Geometry: final body of the model. Coordinates: model frame, mm. Face numbers are marked on the shaded views. A direction names the side the tool comes from. Coordinates: 2 decimals unless noted, no trailing zeros. Write each loop counter-clockwise with the first axis right and the second up, starting at its lowest first coordinate (ties: lowest second). Pieces come first, ordered by that corner, then holes.
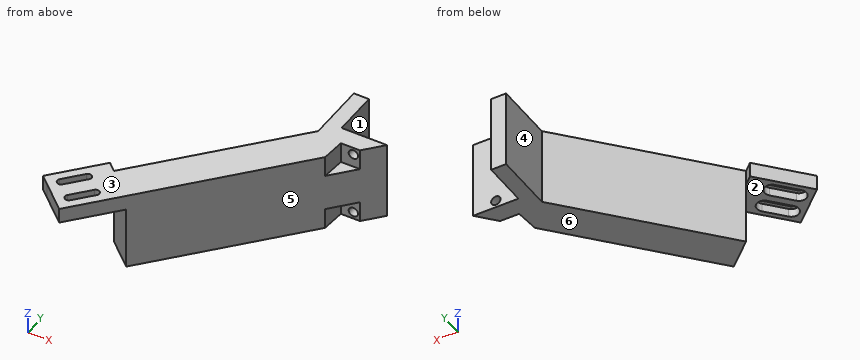
Autodesk Inventor part; units mm, degrees
ref_plane "Work Plane2" through (-4.445, -9.144, -33.02) normal (0, 0, -1) x (0, 1, 0)
ref_plane "YZ Plane" through (0, 0, 0) normal (1, 0, 0) x (0, 1, 0)
ref_plane "XZ Plane" through (0, 0, 0) normal (0, 1, 0) x (-1, 0, 0)
ref_plane "Work Plane1" through (0, 0, 0) normal (0, 0, 1) x (1, 0, 0)
sketch "Sketch1" plane through (0, 0, 0) normal (0, 0, 1) x (1, 0, 0)
  line L0 (4.129202, -9.5377) -> (6.406797, -9.5377) construction
  line L1 (9.525, -8.41296) -> (9.525, -7.435497) construction
  line L2 (-6.406797, 9.5123) -> (-4.129202, 9.5123) construction
  line L3 (-9.525, 4.116502) -> (-9.525, 6.394097) construction
  line L4 (9.314549, -9.373063) -> (-73.965447, -101.864868) construction
  line L5 (9.166309, -9.5377) -> (-73.965447, -101.864868)
  line L6 (-73.965447, -101.864868) -> (-85.121243, -91.820144)
  line L7 (6.33881, 9.756536) -> (-85.121243, -91.820144) construction
  line L8 (9.166309, -9.5377) -> (-9.997679, -9.5377)
  line L9 (-9.997679, -9.5377) -> (-9.997679, 9.756536)
  line L10 (-9.997679, 9.756536) -> (-16.347679, 9.756536)
  line L11 (-16.347679, 9.756536) -> (-16.347679, -15.439362)
  line L12 (-16.347679, -15.439362) -> (-85.121243, -91.820144)
  point P0 (0, 0)
  dimension "d0" = 124.46
  dimension "d1" = 48
  dimension "d5" = 6.35
ref_plane "Work Plane2" through (-4.445, -9.144, -33.02) normal (0, 0, -1) x (0, 1, 0)
extrude "Extrusion1" add sketch "Sketch1" against normal up to surface (33.02 mm away)
sketch "Sketch2" plane through (-73.965447, -101.864868, -33.02) normal (-0.6691306, -0.7431448, 0) x (0.7431448, -0.6691306, 0)
  line L0 (0, 33.02) -> (0, 0)
  line L1 (-15.011605, 33.02) -> (-15.011605, 0)
  line L2 (0, 0) -> (-15.011605, 0)
  line L3 (-15.011605, 0) -> (-15.011605, 26.67)
  line L4 (-15.011605, 26.67) -> (0, 26.67)
  line L5 (0, 26.67) -> (0, 0)
  line L6 (-15.011605, 33.02) -> (0, 33.02)
  point P0 (-13.193862, 33.02)
  dimension "d19" = 6.35
extrude "Extrusion2" cut sketch "Sketch2" against normal blind 25.4 contours L0 L2 L1 L4
sketch "Sketch3" plane through (-73.965447, -101.864868, -6.35) normal (0, 0, -1) x (-0.7431448, 0.6691306, 0)
  line L0 (19.8882, 12.0904) -> (19.8882, 3.175) construction
  line L1 (0, 25.4) -> (15.011605, 25.4) construction
  line L2 (15.011605, 0) -> (0, 0) construction
  line L3 (0, 0) -> (19.8882, 0) construction
  line L4 (19.8882, 0) -> (19.8882, 25.4) construction
  line L5 (19.8882, 25.4) -> (0, 25.4) construction
  line L6 (0, 25.4) -> (0, 0) construction
  line L7 (15.011605, 0) -> (19.8882, 0)
  line L8 (19.8882, 0) -> (19.8882, 25.4)
  line L9 (19.8882, 25.4) -> (15.011605, 25.4)
  line L10 (15.011605, 25.4) -> (15.011605, 0)
  point P0 (13.193862, 125.192894)
extrude "Extrusion3" add sketch "Sketch3" against normal up to surface (6.35 mm away)
sketch "Sketch4" plane through (0, 0, 0) normal (0, 0, 1) x (1, 0, 0)
  line L0 (-88.74526, -88.557064) -> (-71.749342, -69.681186) construction
  line L1 (-73.965447, -101.864868) -> (9.166309, -9.5377) construction
  line L2 (-74.314967, -94.50927) -> (-67.5166, -86.958918) construction
  line L3 (-73.965447, -101.864868) -> (-56.969529, -82.988989) construction
  line L4 (-73.965447, -101.864868) -> (-88.74526, -88.557064) construction
  line L5 (-81.390199, -88.138702) -> (-74.591832, -80.588351) construction
  line L6 (-74.314967, -94.50927) -> (-67.5166, -86.958918) construction
  line L7 (-73.144662, -95.563017) -> (-66.346296, -88.012665)
  line L8 (-68.686904, -85.905171) -> (-75.485271, -93.455523)
  arc A0 (-75.485271, -93.455523) -> (-73.144662, -95.563017) centre (-74.314967, -94.50927) ccw
  arc A1 (-66.346296, -88.012665) -> (-68.686904, -85.905171) centre (-67.5166, -86.958918) ccw
  line L9 (-81.390199, -88.138702) -> (-74.591832, -80.588351) construction
  line L10 (-80.219894, -89.192449) -> (-73.421527, -81.642098)
  line L11 (-75.762136, -79.534604) -> (-82.560503, -87.084955)
  arc A2 (-82.560503, -87.084955) -> (-80.219894, -89.192449) centre (-81.390199, -88.138702) ccw
  arc A3 (-73.421527, -81.642098) -> (-75.762136, -79.534604) centre (-74.591832, -80.588351) ccw
  point P0 (0, 0)
  point P1 (-70.915783, -90.734094)
  point P2 (-77.991015, -84.363527)
  dimension "d37" = 10.16
  dimension "d38" = 5.1816
  dimension "d39" = 5.2324
  dimension "d40" = 9.52066
  dimension "d41" = 3.1496
  dimension "d42" = 3.1496
extrude "Extrusion4" cut sketch "Sketch4" against normal through all
sketch "Sketch6" plane through (-9.997679, -9.5377, 0) normal (0, 1, 0) x (1, 0, 0)
  arc A0 (9.506526, 4.79213) -> (10.740649, 4.300966) centre (9.523849, 3.039616) ccw construction
  arc A1 (9.506526, 31.732899) -> (10.740649, 31.241734) centre (9.523849, 29.980384) ccw construction
  circle A2 centre (9.523849, 29.980384) radius 1.9685
  circle A3 centre (9.523849, 3.039616) radius 1.9685
  point P0 (9.997679, 0)
  dimension "d24" = 3.937
  dimension "d25" = 3.937
extrude "Extrusion6" cut sketch "Sketch6" against normal through all
sketch "Sketch7" plane through (9.166309, -9.5377, 0) normal (0.7431448, -0.6691306, 0) x (0, 0, -1)
  line L0 (33.02, -98.838459) -> (33.02, 0) construction
  line L1 (33.02, -9.525) -> (0, -9.525) construction
  point P0 (0, 0.954435)
sketch "Sketch8" plane through (9.166309, -9.5377, -33.02) normal (0, 0, -1) x (-1, 0, 0)
  line L0 (11.608639, 0) -> (11.608639, -12.892699) construction
  line L1 (66.135838, -73.451289) -> (0, 0) construction
  line L2 (11.608639, -7.62) -> (6.861079, -7.62) construction
  line L3 (0, 0) -> (19.163987, 0) construction
  line L4 (7.671639, 0) -> (7.671639, -8.520218) construction
  line L5 (14.910639, 0) -> (14.910639, -14.251905) construction
  line L6 (6.861079, -7.62) -> (14.910639, -7.62)
  line L7 (83.131755, -92.327168) -> (0, 0)
  line L8 (15.69062, -17.426199) -> (6.861079, -7.62)
  line L9 (15.69062, -17.426199) -> (14.910639, -7.62)
  point P0 (9.166309, 9.5377)
  dimension "d28" = 7.62
  dimension "d29" = 3.302
extrude "Extrusion7" cut sketch "Sketch8" against normal blind 8.763
sketch "Sketch9" plane through (0, 0, 0) normal (0, 0, 1) x (1, 0, 0)
  line L0 (2.30523, -17.1577) -> (-5.74433, -17.1577) construction
  line L1 (-5.74433, -17.1577) -> (-6.524312, -26.963899) construction
  line L2 (2.30523, -17.1577) -> (-6.524312, -26.963899)
  line L3 (-73.965447, -101.864868) -> (9.166309, -9.5377)
  line L4 (2.30523, -17.1577) -> (-5.74433, -17.1577)
  line L5 (-5.2705, -26.963899) -> (-5.2705, -17.1577)
  point P0 (0, 0)
sketch "Sketch9 outline for Extrusion8" plane through (0, 0, 0) normal (0, 0, 1) x (1, 0, 0)
  line L0 (-6.524312, -26.963899) -> (2.30523, -17.1577)
  line L1 (-5.74433, -17.1577) -> (-6.524312, -26.963899)
  line L2 (2.30523, -17.1577) -> (-5.74433, -17.1577)
extrude "Extrusion8" cut sketch "Sketch9 outline for Extrusion8" against normal blind 8.763
sketch "Sketch10" plane through (9.166309, -9.5377, -33.02) normal (0, 0, -1) x (-1, 0, 0)
  line L0 (25.513987, -5.901662) -> (77.291634, -63.406565)
  line L1 (51.797758, -35.092747) -> (40.641962, -45.137471)
  line L2 (66.135838, -73.451289) -> (15.69062, -17.426199) construction
  line L3 (40.913229, -45.438744) -> (36.5125, -40.551239) construction
  line L4 (66.135838, -73.451289) -> (77.291634, -63.406565) construction
  point P0 (9.166309, 9.5377)
  dimension "d34" = 38.1
sketch "Sketch11" plane through (-73.965447, -101.864868, -6.35) normal (0, 0, -1) x (-0.7431448, 0.6691306, 0)
  arc A0 (3.6068, 5.2324) -> (6.7564, 5.2324) centre (5.1816, 5.2324) ccw construction
  arc A1 (6.7564, 15.3924) -> (3.6068, 15.3924) centre (5.1816, 15.3924) ccw construction
  line L0 (5.1816, 5.2324) -> (5.1816, 15.3924) construction
  arc A2 (13.127463, 5.2324) -> (16.277063, 5.2324) centre (14.702263, 5.2324) ccw construction
  arc A3 (16.277063, 15.3924) -> (13.127463, 15.3924) centre (14.702263, 15.3924) ccw construction
  line L1 (14.702263, 5.2324) -> (14.702263, 15.3924) construction
  line L2 (14.702263, 5.2324) -> (14.702263, 15.3924) construction
  line L3 (17.877263, 5.2324) -> (17.877263, 15.3924)
  line L4 (11.527263, 15.3924) -> (11.527263, 5.2324)
  arc A4 (11.527263, 5.2324) -> (17.877263, 5.2324) centre (14.702263, 5.2324) ccw
  arc A5 (17.877263, 15.3924) -> (11.527263, 15.3924) centre (14.702263, 15.3924) ccw
  line L5 (5.1816, 5.2324) -> (5.1816, 15.3924) construction
  line L6 (8.3566, 5.2324) -> (8.3566, 15.3924)
  line L7 (2.0066, 15.3924) -> (2.0066, 5.2324)
  arc A6 (2.0066, 5.2324) -> (8.3566, 5.2324) centre (5.1816, 5.2324) ccw
  arc A7 (8.3566, 15.3924) -> (2.0066, 15.3924) centre (5.1816, 15.3924) ccw
  point P0 (13.193862, 125.192894)
  point P1 (14.702263, 10.3124)
  point P2 (5.1816, 10.3124)
  dimension "d43" = 6.35
  dimension "d44" = 6.35
extrude "Extrusion9" cut sketch "Sketch11" against normal blind 3.556
properties part number "arm stop 48 degree whole"
Item 1: Set-up query: the marked faces 1, 2 and 3. Return all of +Z, -Z, +X, -X, +Y, -Y with unobstructed straight access to the full face (end or side cutting, diameter ignored); none if empty.
Derived:
face 1: +Z, -Z, +X, +Y
face 2: -Z, -X, -Y
face 3: +Z, +X, -X, +Y, -Y
Item 2: Section A-A, the plane z = -13.5. Output: boundary loops of the cut face in (x, y), plus the area to 3 significant figures.
Derived:
outline: (-68.12, -72.94) - (-56.97, -82.99) - (9.17, -9.54) - (-10, -9.54) - (-10, 9.76) - (-16.35, 9.76) - (-16.35, -15.44) - close
area: 1,520 mm2
Item 3: Section D-D, the plane y = -38. Output: boundary loops of the cut face in (x, z), plus the area to 3 significant figures.
Derived:
outline: (-36.66, -33.02) - (-16.46, -33.02) - (-16.46, 0) - (-36.66, 0) - close
area: 667 mm2
Item 4: Pin query (flat end, axial travel): pin 1 (12 mm diameter, centred on y = -2.5, z = -22.5, fed in from -X); pin 2 (4 mm diameter, centred on x = -1.5, z = -4.5, fed in from -Y); pin 3 (1 mm diameter, centred on y = -25.5, z = -27.5, fed in from -X). Return the tip coordinate at first contact, or that it passes through.
Derived:
pin 1: stops at x = -16.35
pin 2: stops at y = -17.16
pin 3: stops at x = -25.86
Item 5: Section C-C, the plane y = -25.5. Output: boundary loops of the cut face in (x, z), plus the area to 3 significant figures.
Derived:
outline: (-25.41, -33.02) - (-6.41, -33.02) - (-6.41, -24.26) - (-5.21, -24.26) - (-5.21, -8.76) - (-6.41, -8.76) - (-6.41, 0) - (-25.41, 0) - close
area: 646 mm2
Item 6: Material intervals for probe 1 along X at (y, z) = (3.5, -5); probe 2 along Z at (x, y) = (-70.5, -95.5); probe 3 along Y at (x, z) = (2, -1.5), sorted ascending.
Derived:
probe 1: x = -16.35 to -10
probe 2: z = -6.35 to 0
probe 3: y = -17.16 to -9.54
Item 7: Section B-B, the plane x = -4. Output: boundary loops of the cut face in (y, z), plus the area to 3 significant figures.
Derived:
outline: (-24.16, -24.26) - (-17.16, -24.26) - (-17.16, -33.02) - (-9.54, -33.02) - (-9.54, 0) - (-17.16, 0) - (-17.16, -8.76) - (-24.16, -8.76) - close
area: 360 mm2
Item 8: Pull-direction query (X, two-part tool) for the marked faces 4, 5 and 6; classes: released by +X, released by -X, zero draft, split by the parting line, or undercut.
Derived:
face 4: released by -X
face 5: released by +X
face 6: zero draft
